Geometry: final body of the model. Coordinates: model frame, mm. Round coordinates to 2 decimals unless told otherwise and drop trailing zeros. Loops run counter-clockwise (first coordinate to the right, second up) from the corner with the lowest first, then second, coordinate; pieces in that order, holes last. Notation, with made-up numbers: (34.25, -23.5) -> (92.25, -23.5) arc R18 cw to (92.25, -15.5) -> close; hole circle Ø1 at (76, 7.25). An arc over 180 degrees is marked (long way). Answer in a Markdown table with one row per item.
```python
from build123d import *

# Parameters (mm, degrees)
SKETCH1_R               = 20
BOSS_EXTRUDE1_DEPTH     = 100
SKETCH2_R               = 15
CUT_EXTRUDE1_DEPTH      = 100
CUT_EXTRUDE5_DEPTH      = 104.923048454
CUT_EXTRUDE5_DEPTH_BACK = 104.923048454
SKETCH6_R               = 2.5


with BuildPart() as part:
    # Sketch1 → Boss-Extrude1 (new body)
    with BuildSketch(Plane.XY):
        Circle(SKETCH1_R)
    extrude(amount=BOSS_EXTRUDE1_DEPTH)

    # Sketch2 → Cut-Extrude1 (cut)
    with BuildSketch(Plane(origin=(0, 0, 0), x_dir=(-1, 0, 0), z_dir=(0, 0, -1))):
        Circle(SKETCH2_R)
    extrude(amount=-CUT_EXTRUDE1_DEPTH, mode=Mode.SUBTRACT)

    # Sketch6 → Cut-Extrude5 (cut, two sides: drawn at the far end of the back side and taken through both)
    with BuildSketch(Plane(origin=(0, 0, 0), x_dir=(0, 0, -1), z_dir=(1, 0, 0)).offset(-CUT_EXTRUDE5_DEPTH_BACK)):
        with Locations((-65.143240637, -0.390136297)):
            Circle(SKETCH6_R)
        with Locations((-35.143240637, -0.390136297)):
            Circle(SKETCH6_R)
    extrude(amount=CUT_EXTRUDE5_DEPTH + CUT_EXTRUDE5_DEPTH_BACK, mode=Mode.SUBTRACT)


solid = part.part
```
Item 1: Section query B-B, the plane y = 8.5. Output: boundary loops of the cut face in (x, z).
Ans:
| item | result |
|---|---|
| outline | (-18.1, 0) -> (-12.36, 0) -> (-12.36, 100) -> (-18.1, 100) -> close; (12.36, 0) -> (18.1, 0) -> (18.1, 100) -> (12.36, 100) -> close |
Item 2: Section query A-A, the plane x = -12. Output: boundary loops of the cut face in (y, z), and give its area (3 significant figures).
Ans:
| item | result |
|---|---|
| outline | (-16, 0) -> (-9, 0) -> (-9, 100) -> (-16, 100) -> close; (9, 0) -> (16, 0) -> (16, 100) -> (9, 100) -> close |
| area | 1,400 mm2 |
Item 3: Mould query, pull axis Z, two halves, no side actions, for faces 1 (the flat face through (3, 15, 0)), 2 (the cylindrical face through (17.32, -2.83, 65.69)), 3 (the flat face through (3, 15, 100)). Classes: released by +Z, released by -Z, zero draft, split by the parting line, or undercut.
Ans:
| item | result |
|---|---|
| face 1 | released by -Z |
| face 2 | undercut |
| face 3 | released by +Z |
Item 4: Ray query, L1, parallel to X at y = 0, z = 32; L2, parallel to Y at x = -3, z = 93.5; L3, parallel to Y at x = 4.5, z = 95.5. Return the intervals inside material, ascending.
Ans:
| item | result |
|---|---|
| L1 | -20 to -15, 15 to 20 |
| L2 | -19.77 to -14.7, 14.7 to 19.77 |
| L3 | -19.49 to -14.31, 14.31 to 19.49 |
Item 5: Section query C-C, the plane z = 93.5. Output: boundary loops of the cut face in (x, y).
Ans:
| item | result |
|---|---|
| outline | circle Ø40 at (0, 0); hole circle Ø30 at (0, 0) |
Item 6: Section query D-D, the plane x = 17. Output: boundary loops of the cut face in (y, z).
Ans:
| item | result |
|---|---|
| outline | (-10.54, 0) -> (10.54, 0) -> (10.54, 100) -> (-10.54, 100) -> close; hole circle Ø5 at (-0.39, 35.14); hole circle Ø5 at (-0.39, 65.14) |
Item 7: First-contact query: P1, Ø24, axis at x = 0, y = 0, coming from the -Z side; P2, Ø1.5, axis at y = -11.5, z = 87, coming from the +X side; P3, Ø2, axis at y = 4, z = 70.5, coming from the +X side; P4, Ø3, axis at y = 5.5, z = 47.5, coming from the -X side. Flat tips, straight axial feed; report the tip coordinate or a pass-through.
Ans:
| item | result |
|---|---|
| P1 | through |
| P2 | x = 16.87 |
| P3 | x = 19.77 |
| P4 | x = -19.6 |
